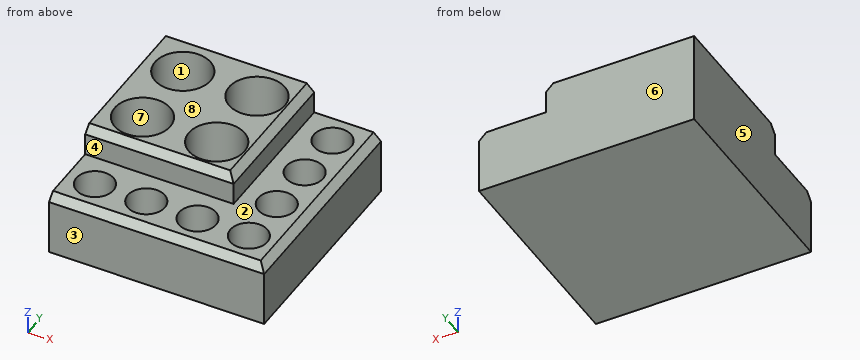
from build123d import *

# Parameters (mm, degrees)
F0_R     = 7.5
F1_DEPTH = 25
F0_R_2   = 5
F2_DEPTH = 17
F3_DEPTH = 3
F4_SIZE  = 2


with BuildPart() as f1:
    # F0 (on Top) → F1 (new body)
    with BuildSketch(Plane.XY):
        Polygon((20, 0), (0, 0), (0, -20), (0, -40), (40, -40), (40, 0), align=None)
        with Locations((10, -30)):
            Circle(F0_R, mode=Mode.SUBTRACT)
        with Locations((30, -30)):
            Circle(F0_R, mode=Mode.SUBTRACT)
        with Locations((10, -10)):
            Circle(F0_R, mode=Mode.SUBTRACT)
        with Locations((30, -10)):
            Circle(F0_R, mode=Mode.SUBTRACT)
    extrude(amount=F1_DEPTH)

    # F0 (on Top) → F2 (join)
    with BuildSketch(Plane.XY):
        Polygon((58, 0), (40, 0), (40, -40), (0, -40), (0, -58), (58, -58), align=None)
        with Locations((7.5, -49)):
            Circle(F0_R_2, mode=Mode.SUBTRACT)
        with Locations((21.333333, -49)):
            Circle(F0_R_2, mode=Mode.SUBTRACT)
        with Locations((35.166667, -49)):
            Circle(F0_R_2, mode=Mode.SUBTRACT)
        with Locations((49, -49)):
            Circle(F0_R_2, mode=Mode.SUBTRACT)
        with Locations((49, -35.166667)):
            Circle(F0_R_2, mode=Mode.SUBTRACT)
        with Locations((49, -21.333333)):
            Circle(F0_R_2, mode=Mode.SUBTRACT)
        with Locations((49, -7.5)):
            Circle(F0_R_2, mode=Mode.SUBTRACT)
    extrude(amount=F2_DEPTH)

    # F0 (on Top) → F3 (join)
    with BuildSketch(Plane.XY):
        with Locations((10, -10)):
            Circle(F0_R)
        with Locations((30, -10)):
            Circle(F0_R)
        with Locations((30, -30)):
            Circle(F0_R)
        with Locations((10, -30)):
            Circle(F0_R)
        with Locations((7.5, -49)):
            Circle(F0_R_2)
        with Locations((21.333333, -49)):
            Circle(F0_R_2)
        with Locations((35.166667, -49)):
            Circle(F0_R_2)
        with Locations((49, -49)):
            Circle(F0_R_2)
        with Locations((49, -35.166667)):
            Circle(F0_R_2)
        with Locations((49, -21.333333)):
            Circle(F0_R_2)
        with Locations((49, -7.5)):
            Circle(F0_R_2)
    extrude(amount=F3_DEPTH)

    # F4
    f4_edges = [f1.edges().sort_by_distance(p)[0] for p in [
        (20, -40, 25),
        (40, -20, 25),
        (29, -58, 17),
        (58, -29, 17),
    ]]
    chamfer(f4_edges, length=F4_SIZE)


solid = f1.part
Verification items for the finished model (mm, model axes). Face numbers are marked on the shaded views. A direction names the side the tool comes from. Coordinates: 2 decimals unless noted, no trailing zeros. Order: outer loops, then holes, each group sorted by start corner. A loop starts at its lowest first (then second) coordinate and runs counter-clockwise, first axis right, second up.
1. Sectioned sample at C-C, the plane z = 16.25. Give the number of separate pieces and of enclosed holes in the cut face, and give its area (3 significant figures).
Results found:
separate pieces: 1
enclosed holes: 11
area: 1,960 mm2
2. Sectioned sample at D-D, the plane y = -31. Record the cut outline in (x, z), and give its area (3 significant figures).
Results found:
outline: (0, 0) - (58, 0) - (58, 15) - (56, 17) - (51.76, 17) - (51.76, 3) - (46.24, 3) - (46.24, 17) - (40, 17) - (40, 23) - (38, 25) - (37.43, 25) - (37.43, 3) - (22.57, 3) - (22.57, 25) - (17.43, 25) - (17.43, 3) - (2.57, 3) - (2.57, 25) - (0, 25) - close
area: 571 mm2
3. Sectioned sample at B-B, the plane x = 11. Record the cut outline in (y, z).
Results found:
outline: (-58, 0) - (0, 0) - (0, 25) - (-2.57, 25) - (-2.57, 3) - (-17.43, 3) - (-17.43, 25) - (-22.57, 25) - (-22.57, 3) - (-37.43, 3) - (-37.43, 25) - (-38, 25) - (-40, 23) - (-40, 17) - (-45.43, 17) - (-45.43, 3) - (-52.57, 3) - (-52.57, 17) - (-56, 17) - (-58, 15) - close
4. Release check for a two-part mould opening along Y. For the marked faces 6, 7 and 8 record: +Y half, -Y half, draft (parallel to the pull), parting line (faces both ways), or undercut.
Results found:
face 6: +Y half
face 7: undercut
face 8: draft
5. Scan lines: line 1 (Y direction, x = 30, z = 21.75); line 2 (Y direction, x = 49, z = 14.25); line 3 (Y direction, x = 30, z = 10). Record each from-to range of solid material in increasing order.
Results found:
line 1: y = -40 to -37.5, -22.5 to -17.5, -2.5 to 0
line 2: y = -58 to -54, -44 to -40.17, -30.17 to -26.33, -16.33 to -12.5, -2.5 to 0
line 3: y = -58 to -37.5, -22.5 to -17.5, -2.5 to 0
6. Go/stop test with flat-tipped pins: pin 1 Ø1 at (x, z) = (16.5, 17) entering from -Y; pin 2 Ø4.5 at (x, y) = (31.5, -31) entering from +Z; pin 3 Ø3 at (x, z) = (11, 19) entering from -Y. Record where each tip stops, or that it passes through.
Results found:
pin 1: stops at y = -56.5
pin 2: stops at z = 3
pin 3: stops at y = -40
7. Sectioned sample at A-A, the plane y = -49. Record the cut outline in (x, z).
Results found:
outline: (0, 0) - (58, 0) - (58, 15) - (56, 17) - (54, 17) - (54, 3) - (44, 3) - (44, 17) - (40.17, 17) - (40.17, 3) - (30.17, 3) - (30.17, 17) - (26.33, 17) - (26.33, 3) - (16.33, 3) - (16.33, 17) - (12.5, 17) - (12.5, 3) - (2.5, 3) - (2.5, 17) - (0, 17) - close
8. Set-up check for the marked faces 1, 2, 3, 4 and 5: record each of +Z, -Z, +X, -X, +Y, -Y from which the full face is reachable in a straight line by a thin tool's end or side.
Results found:
face 1: +Z
face 2: +Z, +X, -Y
face 3: +Z, -Z, +X, -X, -Y
face 4: +Z, +X, -X, -Y
face 5: +Z, -Z, -X, +Y, -Y
